Can you work these out from the model? Positions are in its coordinate system, mm. Give positions to 0.01 mm unless a question says otherwise; leave off trailing zeros. Order: outer loops, then holes, each group sorted by start corner. A loop starts at its lowest first (then second) coordinate and runs counter-clockwise, first axis right, second up. Notation, with made-up numbers: (64, 78) - (73, 78) arc R24 ccw to (73, 109) - close; hole circle Ø1 at (-12.75, 63). An arc over 180 degrees is marked (long way). Answer as a JSON object with one key per item and string values.
```python
from build123d import *

# Parameters (mm, degrees)
ESQUISSE1_W             = 100
ESQUISSE1_H             = 35
BOSS_EXTRU_1_DEPTH      = 3
ESQUISSE2_R             = 1.5
ENL_V_MAT_EXTRU_1_DEPTH = 3
CONG_1_R                = 1


with BuildPart() as part:
    # Esquisse1 → Boss.-Extru.1 (new body)
    with BuildSketch(Plane.XY):
        with Locations((50, 17.5)):
            Rectangle(ESQUISSE1_W, ESQUISSE1_H)
    extrude(amount=BOSS_EXTRU_1_DEPTH)

    # Esquisse2 → Enlèv. mat.-Extru.1 (cut)
    with BuildSketch(Plane.XY.offset(3)):
        with Locations((95, 32.5)):
            Circle(ESQUISSE2_R)
        with Locations((85, 32.5)):
            Circle(ESQUISSE2_R)
        with Locations((75, 32.5)):
            Circle(ESQUISSE2_R)
        with Locations((65, 32.5)):
            Circle(ESQUISSE2_R)
        with Locations((55, 32.5)):
            Circle(ESQUISSE2_R)
        with Locations((45, 32.5)):
            Circle(ESQUISSE2_R)
        with Locations((35, 32.5)):
            Circle(ESQUISSE2_R)
        with Locations((25, 32.5)):
            Circle(ESQUISSE2_R)
        with Locations((15, 32.5)):
            Circle(ESQUISSE2_R)
        with Locations((5, 32.5)):
            Circle(ESQUISSE2_R)
        with Locations((85, 22.5)):
            Circle(ESQUISSE2_R)
        with Locations((75, 22.5)):
            Circle(ESQUISSE2_R)
        with Locations((65, 22.5)):
            Circle(ESQUISSE2_R)
        with Locations((55, 22.5)):
            Circle(ESQUISSE2_R)
        with Locations((45, 22.5)):
            Circle(ESQUISSE2_R)
        with Locations((35, 22.5)):
            Circle(ESQUISSE2_R)
        with Locations((25, 22.5)):
            Circle(ESQUISSE2_R)
        with Locations((15, 22.5)):
            Circle(ESQUISSE2_R)
        with Locations((5, 22.5)):
            Circle(ESQUISSE2_R)
        with Locations((85, 12.5)):
            Circle(ESQUISSE2_R)
        with Locations((75, 12.5)):
            Circle(ESQUISSE2_R)
        with Locations((65, 12.5)):
            Circle(ESQUISSE2_R)
        with Locations((55, 12.5)):
            Circle(ESQUISSE2_R)
        with Locations((45, 12.5)):
            Circle(ESQUISSE2_R)
        with Locations((35, 12.5)):
            Circle(ESQUISSE2_R)
        with Locations((25, 12.5)):
            Circle(ESQUISSE2_R)
        with Locations((15, 12.5)):
            Circle(ESQUISSE2_R)
        with Locations((5, 12.5)):
            Circle(ESQUISSE2_R)
        with Locations((85, 2.5)):
            Circle(ESQUISSE2_R)
        with Locations((75, 2.5)):
            Circle(ESQUISSE2_R)
        with Locations((65, 2.5)):
            Circle(ESQUISSE2_R)
        with Locations((55, 2.5)):
            Circle(ESQUISSE2_R)
        with Locations((45, 2.5)):
            Circle(ESQUISSE2_R)
        with Locations((35, 2.5)):
            Circle(ESQUISSE2_R)
        with Locations((25, 2.5)):
            Circle(ESQUISSE2_R)
        with Locations((15, 2.5)):
            Circle(ESQUISSE2_R)
        with Locations((5, 2.5)):
            Circle(ESQUISSE2_R)
        with Locations((95, 22.5)):
            Circle(ESQUISSE2_R)
        with Locations((95, 12.5)):
            Circle(ESQUISSE2_R)
        with Locations((95, 2.5)):
            Circle(ESQUISSE2_R)
    extrude(amount=-ENL_V_MAT_EXTRU_1_DEPTH, mode=Mode.SUBTRACT)

    # Congé1
    cong_1_edges = [part.edges().sort_by_distance(p)[0] for p in [
        (0, 35, 1.5),
        (100, 35, 1.5),
        (100, 0, 1.5),
        (0, 0, 1.5),
    ]]
    fillet(cong_1_edges, radius=CONG_1_R)


solid = part.part
```
Q1. If we section it at B-B, the plane z = 1.55: Count the separate pieces of the cut face and the enclosed holes in it, then the cut area to 3 significant figures.
Recorded:
{"separate pieces": "1", "enclosed holes": "40", "area": "3,220 mm^2"}
Q2. I need wall thicknesses on L1, parallel to Y at x = 45, z = 1.5; L2, parallel to Y at x = 55.5, z = 1.7. Which ranges of each line are inside material? Lowest first, please.
Recorded:
{"L1": "y = 0 to 1, 4 to 11, 14 to 21, 24 to 31, 34 to 35", "L2": "y = 0 to 1.09, 3.91 to 11.09, 13.91 to 21.09, 23.91 to 31.09, 33.91 to 35"}
Q3. We'd pull the mould along X, two halves only. Please class faces 1 (the face through (66.43, 22.95, 1.52)), 2 (the face through (0, 17, 1)): released by +X, released by -X, zero draft, split by the parting line, or undercut.
Recorded:
{"face 1": "undercut", "face 2": "released by -X"}
Q4. If we section it at A-A, the plane x = 85: Please give me the cut outline in (y, z), then the cut area to 3 significant figures.
Recorded:
{"outline": "(0, 0) - (1, 0) - (1, 3) - (0, 3) - close; (4, 0) - (11, 0) - (11, 3) - (4, 3) - close; (14, 0) - (21, 0) - (21, 3) - (14, 3) - close; (24, 0) - (31, 0) - (31, 3) - (24, 3) - close; (34, 0) - (35, 0) - (35, 3) - (34, 3) - close", "area": "69.0 mm^2"}
